Can you work these out from the model? Positions are in its coordinate system, mm. Face numbers are marked on the shaded views. Round coordinates to 2 decimals unless told otherwise and drop trailing zeros. Loops run counter-clockwise (first coordinate to the right, second up) from the corner with the lowest first, then second, coordinate; pieces in that order, holes last. Notation, with made-up numbers: (42.5, 8) -> (91.5, 8) arc R6 cw to (91.5, 13) -> close; hole circle Ø10 at (75.5, 17). An arc over 180 degrees is marked (long way). Use a Markdown table: item, result.
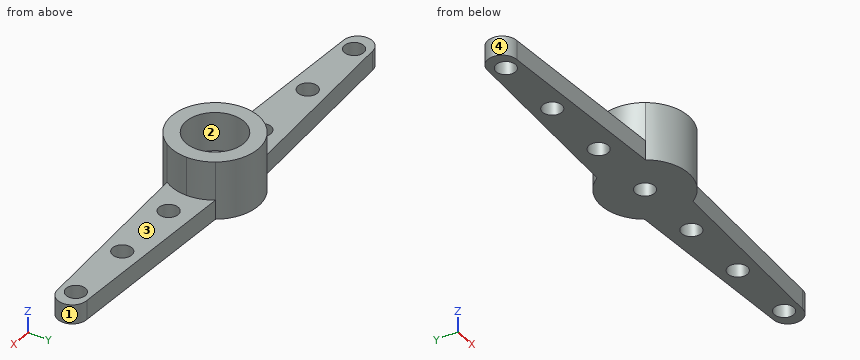
from build123d import *

# Parameters (mm, degrees)
SKETCH1_R           = 1.5
SKETCH1_R_2         = 4.5
BOSS_EXTRUDE1_DEPTH = 6
CUT_EXTRUDE1_START  = -4
SKETCH3_R           = 3
CUT_EXTRUDE1_DEPTH  = 4
SKETCH4_R           = 1
CUT_EXTRUDE2_DEPTH  = 10


with BuildPart() as part:
    # Sketch1 → Boss-Extrude1 (new body)
    with BuildSketch(Plane.XY):
        with Locations((-22.5, 0)):
            Circle(SKETCH1_R)
        with BuildLine():
            Line((-3.75, 2.487468593), (-22.5, 1.5))
            ThreePointArc((-22.5, 1.5), (-21.439339828, 1.060660172), (-21, 0))
            ThreePointArc((-21, 0), (-21.439339828, -1.060660172), (-22.5, -1.5))
            Line((-22.5, -1.5), (-3.75, -2.487468593))
            ThreePointArc((-3.75, -2.487468593), (-4.5, 0), (-3.75, 2.487468593))
        make_face()
        Circle(SKETCH1_R_2)
        with BuildLine():
            ThreePointArc((22.5, -1.5), (21, 0), (22.5, 1.5))
            Line((22.5, 1.5), (3.75, 2.487468593))
            ThreePointArc((3.75, 2.487468593), (4.308421985, 1.299038106), (4.5, 0))
            ThreePointArc((4.5, 0), (4.308421985, -1.299038106), (3.75, -2.487468593))
            Line((3.75, -2.487468593), (22.5, -1.5))
        make_face()
        with Locations((22.5, 0)):
            Circle(SKETCH1_R)
    extrude(amount=BOSS_EXTRUDE1_DEPTH)

    # Sketch3 → Cut-Extrude1 (cut)
    with BuildSketch(Plane.XY.offset(6).offset(CUT_EXTRUDE1_START)):
        with BuildLine():
            ThreePointArc((-22.5, 1.5), (-24, 0), (-22.5, -1.5))
            Line((-22.5, -1.5), (-3.75, -2.487468593))
            ThreePointArc((-3.75, -2.487468593), (-4.5, 0), (-3.75, 2.487468593))
            Line((-3.75, 2.487468593), (-22.5, 1.5))
        make_face()
        with BuildLine():
            ThreePointArc((4.5, 0), (4.308421985, -1.299038106), (3.75, -2.487468593))
            Line((3.75, -2.487468593), (22.5, -1.5))
            ThreePointArc((22.5, -1.5), (24, 0), (22.5, 1.5))
            Line((22.5, 1.5), (3.75, 2.487468593))
            ThreePointArc((3.75, 2.487468593), (4.308421985, 1.299038106), (4.5, 0))
        make_face()
        Circle(SKETCH3_R)
    extrude(amount=CUT_EXTRUDE1_DEPTH, mode=Mode.SUBTRACT)

    # Sketch4 → Cut-Extrude2 (cut)
    with BuildSketch(Plane(origin=(0, 0, 0), x_dir=(-1, 0, 0), z_dir=(0, 0, -1))):
        Circle(SKETCH4_R)
        with Locations((7.312902248, 0)):
            Circle(SKETCH4_R)
        with Locations((14.625804497, 0)):
            Circle(SKETCH4_R)
        with Locations((21.938706745, 0)):
            Circle(SKETCH4_R)
    cut_extrude2 = extrude(amount=-CUT_EXTRUDE2_DEPTH, mode=Mode.SUBTRACT)

    # Mirror1: Cut-Extrude2 across plane
    add(cut_extrude2.mirror(Plane(origin=(0, 0, 0), x_dir=(0, 0, 1), z_dir=(1, 0, 0))), mode=Mode.SUBTRACT)


solid = part.part
1. Will these pins go through, and if not, where does the flat tip stop? pin 1 Ø1.5 at (x, z) = (12, 4) entering from -Y; pin 2 Ø3 at (x, y) = (-7.31, 0) entering from +Z; pin 3 Ø3 at (x, z) = (-7.5, 1) entering from +Y; pin 4 Ø2 at (x, z) = (-18.5, 2.5) entering from +Y.
Answer sheet:
| item | result |
|---|---|
| pin 1 | passes through |
| pin 2 | stops at z = 2 |
| pin 3 | stops at y = 2.37 |
| pin 4 | stops at y = 1.76 |
2. If we mould it in two halves opening along X, with no side actions, what happens to the marked faces 1, 2, 3 and 4? For each: +X half, -X half, draft (parallel to the pull), parting line (faces both ways), or undercut.
Answer sheet:
| item | result |
|---|---|
| face 1 | +X half |
| face 2 | undercut |
| face 3 | draft |
| face 4 | -X half |
3. I want a section at C-C (y = -2). Please give me the cut outline in (x, z), plus the area to 3 significant figures.
Answer sheet:
| item | result |
|---|---|
| outline | (-13.01, 0) -> (13.01, 0) -> (13.01, 2) -> (4.03, 2) -> (4.03, 6) -> (2.24, 6) -> (2.24, 2) -> (-2.24, 2) -> (-2.24, 6) -> (-4.03, 6) -> (-4.03, 2) -> (-13.01, 2) -> close |
| area | 66.4 mm² |
4. I want a section at D-D (x = 5.5). Please give me the cut outline in (y, z), plus the area to 3 significant figures.
Answer sheet:
| item | result |
|---|---|
| outline | (-2.4, 0) -> (2.4, 0) -> (2.4, 2) -> (-2.4, 2) -> close |
| area | 9.58 mm² |
5. I want a section at A-A (x = 0). Please give me the cut outline in (y, z), plus the area to 3 significant figures.
Answer sheet:
| item | result |
|---|---|
| outline | (-4.5, 0) -> (-1, 0) -> (-1, 2) -> (-3, 2) -> (-3, 6) -> (-4.5, 6) -> close; (1, 0) -> (4.5, 0) -> (4.5, 6) -> (3, 6) -> (3, 2) -> (1, 2) -> close |
| area | 26.0 mm² |
6. I need wall thicknesses on line 1 (Z direction, x = 20, y = 1); line 2 (Y direction, x = -1, z = 2.85); line 3 (Y direction, x = -6.5, z = 1.1). Which ranges of each line are inside material? Lowest first, please.
Answer sheet:
| item | result |
|---|---|
| line 1 | z = 0 to 2 |
| line 2 | y = -4.39 to -2.83, 2.83 to 4.39 |
| line 3 | y = -2.34 to -0.58, 0.58 to 2.34 |
7. I want a section at B-B (z = 4.1). Please give me the cut outline in (x, y).
Answer sheet:
| item | result |
|---|---|
| outline | circle Ø9 at (0, 0); hole circle Ø6 at (0, 0) |
